Check sheet for the modelled part. Datum: model origin and axes. Units: mm. A direction names the side the tool comes from. Round coordinates to 2 decimals unless told otherwise and drop trailing zeros. Write each loop counter-clockwise with the first axis right and the second up, starting at its lowest first coordinate (ties: lowest second). Pieces come first, ordered by that corner, then holes. Notation, with made-up numbers: (60, 86) - (78, 86) arc R17 ccw to (78, 94) - close; hole circle Ø7 at (30, -13.5). An arc over 180 degrees is marked (long way). Answer as a JSON object with one key per item and string values. Group by question number.
Item 1: Thickness scan on line 1 (Z direction, x = 2.75, y = 73.66) (3 decimals); line 2 (X direction, y = 46, z = -1); line 3 (X direction, y = 39.5, z = 38.5). Record the ranges inside material, lowest first.
Item 2: Gauge pin test, flat ends, axial feed: P1, Ø1.3, axis at x = 1.5, z = -4, coming from the +Y side; P2, Ø5, axis at y = 69.5, z = -1, coming from the +X side; P3, Ø2, axis at x = 1.5, z = 21.5, coming from the +Y side. Record the tip position at first contact, or that the pin passes through.
Item 3: Set-up check for faces 1 (the flat face through (1, 44.45, -28)), 2 (the cylindrical face through (5.633, 81.215, 21.868)): record each of +Z, -Z, +X, -X, +Y, -Y from which the full face is reachable in a straight line by a thin tool's end or side.
Item 4: Sectioned sample at A-A on y = 73.66. Record the boundary of the cut face in (x, z) (3 decimals), plus the area to 3 significant figures.
Item 5: Sectioned sample at B-B on z = 18.5. Record the boundary of the cut face in (x, y).
Item 6: Release check for a two-part mould opening along Z. For faces 3 (the flat face through (5, 63, 50.8)), 4 (the flat face through (6.95, 100.99, 0.71)), 5 (the flat face through (1, 42, 13.511)) record: pulls with the +Z half, pulls with the -Z half, needs draft (parallel to the pull), parting line crosses it, or undercut.
Item 7: Sectioned sample at C-C on x = 6. Record the boundary of the cut face in (y, z) (3 decimals).
Item 8: Sectioned sample at D-D on z = 36. Record the boundary of the cut face in (x, y), plus the area to 3 significant figures.
Autodesk Inventor part; units mm, degrees
ref_plane "YZ Plane" through (0, 0, 0) normal (1, 0, 0) x (0, 1, 0)
ref_plane "XZ Plane" through (0, 0, 0) normal (0, 1, 0) x (-1, 0, 0)
sketch "Sketch1" plane through (0, 0, 0) normal (0, 0, 1) x (1, 0, 0)
  line L0 (0, 0) -> (14.2789, 101.6)
  line L1 (14.2789, 101.6) -> (0, 101.6)
  line L2 (0, 101.6) -> (0, 0)
  dimension "d0" = 101.6
  dimension "d1" = 8
  dimension "d2" = 14.279
extrude "Extrusion1" add sketch "Sketch1" along normal mid plane 101.6
ref_plane "Work Plane2" through (0, 0, 42.3872) normal (-1, 0, 0) x (0, 0, 1)
sketch "Sketch6" plane through (0, 0, 42.3872) normal (-1, 0, 0) x (0, 0, 1)
  line L0 (-84.1061, 73.66) -> (0, 73.66) construction
  line L1 (0, 101.6) -> (0, 0) construction
  line L2 (-84.7743, 101.6) -> (0, 101.6) construction
  circle A0 centre (-65.2472, 73.66) radius 9.525
  circle A1 centre (-19.5272, 73.66) radius 7.62
  line L3 (-42.3872, 121.92) -> (-42.3872, -20.32)
  point P0 (-42.3872, 0)
  dimension "d18" = 27.94
  dimension "d19" = 19.05
  dimension "d20" = 15.24
  dimension "d21" = 22.86
  dimension "d22" = 22.86
  dimension "d23" = 45.72
extrude "Extrusion5" cut sketch "Sketch6" against normal through all
ref_plane "Work Plane3" through (0, 0, 22.86) normal (0, 0, 1) x (1, 0, 0)
ref_plane "Work Plane4" through (0, 0, -22.86) normal (0, 0, 1) x (1, 0, 0)
sketch "Sketch9" plane through (0, 0, -50.8) normal (-1, 0, 0) x (0, 0, 1)
  line L0 (0, 101.6) -> (0, 0) construction
  line L1 (0, 38.1) -> (100.9997, 38.1) construction
  line L2 (0, 0) -> (101.6, 0) construction
  spline S0 degree 2 poles (30.4104, 35.6403) (30.4104, 34.6934) (29.6899, 33.2629) (29.093, 32.7895) knots 0 0 0 1 2 2 2
  spline S1 degree 2 poles (29.093, 32.7895) (28.3726, 32.2234) (26.6642, 31.75) (25.3365, 31.75) knots 0 0 0 1 2 2 2
  line L3 (25.3365, 31.75) -> (20.2627, 31.75)
  line L4 (20.2627, 31.75) -> (20.2627, 44.45)
  line L5 (20.2627, 44.45) -> (24.7396, 44.45)
  spline S2 degree 2 poles (24.7396, 44.45) (26.1393, 44.45) (27.5801, 44.2339) (28.2079, 43.8942) knots 0 0 0 1 2 2 2
  spline S3 degree 2 poles (28.2079, 43.8942) (28.8975, 43.534) (29.5664, 42.299) (29.5664, 41.4963) knots 0 0 0 1 2 2 2
  spline S4 degree 2 poles (29.5664, 41.4963) (29.5664, 40.57) (28.6402, 39.1189) (27.8169, 38.7793) knots 0 0 0 1 2 2 2
  line L6 (27.8169, 38.7793) -> (27.8169, 38.7175)
  spline S5 degree 2 poles (27.8169, 38.7175) (29.0004, 38.4705) (30.4104, 36.937) (30.4104, 35.6403) knots 0 0 0 1 2 2 2
  spline S6 degree 2 poles (27.117, 35.6917) (27.117, 36.2887) (26.6436, 36.9576) (26.1702, 37.1326) knots 0 0 0 1 2 2 2
  spline S7 degree 2 poles (26.1702, 37.1326) (25.882, 37.2458) (24.8631, 37.2664) (24.0192, 37.2664) knots 0 0 0 1 2 2 2
  line L7 (24.0192, 37.2664) -> (23.4326, 37.2664)
  line L8 (23.4326, 37.2664) -> (23.4326, 34.0656)
  line L9 (23.4326, 34.0656) -> (23.6075, 34.0656)
  spline S8 degree 2 poles (23.6075, 34.0656) (24.8425, 34.0656) (25.7894, 34.0965) (26.2834, 34.3126) knots 0 0 0 1 2 2 2
  spline S9 degree 2 poles (26.2834, 34.3126) (26.7156, 34.5082) (27.117, 35.2286) (27.117, 35.6917) knots 0 0 0 1 2 2 2
  spline S10 degree 2 poles (26.3246, 40.8685) (26.3246, 41.1772) (26.0055, 41.8256) (25.6762, 41.9697) knots 0 0 0 1 2 2 2
  spline S11 degree 2 poles (25.6762, 41.9697) (25.3674, 42.1138) (24.5029, 42.1344) (23.6487, 42.1344) knots 0 0 0 1 2 2 2
  line L10 (23.6487, 42.1344) -> (23.4326, 42.1344)
  line L11 (23.4326, 42.1344) -> (23.4326, 39.4379)
  line L12 (23.4326, 39.4379) -> (23.834, 39.4379)
  spline S12 degree 2 poles (23.834, 39.4379) (24.647, 39.4379) (25.3057, 39.4688) (25.6556, 39.6335) knots 0 0 0 1 2 2 2
  spline S13 degree 2 poles (25.6556, 39.6335) (26.0364, 39.8187) (26.3246, 40.4465) (26.3246, 40.8685) knots 0 0 0 1 2 2 2
  line L13 (35.9885, 31.75) -> (40.2801, 44.45)
  line L14 (40.2801, 44.45) -> (43.7587, 44.45)
  line L15 (43.7587, 44.45) -> (48.0504, 31.75)
  line L16 (48.0504, 31.75) -> (44.7673, 31.75)
  line L17 (44.7673, 31.75) -> (43.9749, 34.3435)
  line L18 (43.9749, 34.3435) -> (39.9817, 34.3435)
  line L19 (39.9817, 34.3435) -> (39.1789, 31.75)
  line L20 (39.1789, 31.75) -> (35.9885, 31.75)
  line L21 (43.275, 36.6489) -> (41.9783, 40.8479)
  line L22 (41.9783, 40.8479) -> (40.6712, 36.6489)
  line L23 (40.6712, 36.6489) -> (43.275, 36.6489)
  spline S14 degree 2 poles (60.0094, 31.503) (57.1483, 31.503) (53.7932, 34.961) (53.7932, 38.0897) knots 0 0 0 1 2 2 2
  spline S15 degree 2 poles (53.7932, 38.0897) (53.7932, 41.1052) (57.1586, 44.697) (60.0197, 44.697) knots 0 0 0 1 2 2 2
  spline S16 degree 2 poles (60.0197, 44.697) (60.771, 44.697) (61.9854, 44.522) (62.5412, 44.378) knots 0 0 0 1 2 2 2
  spline S17 degree 2 poles (62.5412, 44.378) (62.9734, 44.2442) (63.9923, 43.8016) (64.3113, 43.637) knots 0 0 0 1 2 2 2
  line L24 (64.3113, 43.637) -> (64.3113, 40.6112)
  line L25 (64.3113, 40.6112) -> (63.9923, 40.6112)
  spline S18 degree 2 poles (63.9923, 40.6112) (63.7556, 40.817) (63.0557, 41.3934) (62.6132, 41.6609) knots 0 0 0 1 2 2 2
  spline S19 degree 2 poles (62.6132, 41.6609) (62.1707, 41.9388) (61.1106, 42.3196) (60.524, 42.3196) knots 0 0 0 1 2 2 2
  spline S20 degree 2 poles (60.524, 42.3196) (59.8344, 42.3196) (58.6921, 41.8874) (58.1672, 41.3419) knots 0 0 0 1 2 2 2
  spline S21 degree 2 poles (58.1672, 41.3419) (57.6938, 40.8582) (57.0865, 39.2012) (57.0865, 38.0794) knots 0 0 0 1 2 2 2
  spline S22 degree 2 poles (57.0865, 38.0794) (57.0865, 36.8959) (57.7143, 35.2801) (58.2289, 34.7861) knots 0 0 0 1 2 2 2
  spline S23 degree 2 poles (58.2289, 34.7861) (58.7229, 34.3024) (59.9374, 33.8804) (60.5446, 33.8804) knots 0 0 0 1 2 2 2
  spline S24 degree 2 poles (60.5446, 33.8804) (61.1724, 33.8804) (62.3147, 34.3024) (62.7058, 34.5596) knots 0 0 0 1 2 2 2
  spline S25 degree 2 poles (62.7058, 34.5596) (63.1381, 34.8169) (63.7865, 35.3624) (64.0232, 35.5785) knots 0 0 0 1 2 2 2
  line L26 (64.0232, 35.5785) -> (64.3113, 35.5785)
  line L27 (64.3113, 35.5785) -> (64.3113, 32.5939)
  spline S26 degree 2 poles (64.3113, 32.5939) (63.9614, 32.4293) (63.0455, 32.0176) (62.5515, 31.8735) knots 0 0 0 1 2 2 2
  spline S27 degree 2 poles (62.5515, 31.8735) (61.9545, 31.6882) (60.9151, 31.503) (60.0094, 31.503) knots 0 0 0 1 2 2 2
  line L28 (82.4351, 31.75) -> (78.5757, 31.75)
  line L29 (78.5757, 31.75) -> (75.128, 36.9062)
  line L30 (75.128, 36.9062) -> (74.5002, 36.0417)
  line L31 (74.5002, 36.0417) -> (74.5002, 31.75)
  line L32 (74.5002, 31.75) -> (71.3097, 31.75)
  line L33 (71.3097, 31.75) -> (71.3097, 44.45)
  line L34 (71.3097, 44.45) -> (74.5002, 44.45)
  line L35 (74.5002, 44.45) -> (74.5002, 38.7793)
  line L36 (74.5002, 38.7793) -> (78.5757, 44.45)
  line L37 (78.5757, 44.45) -> (82.2498, 44.45)
  line L38 (82.2498, 44.45) -> (77.7215, 38.5528)
  line L39 (77.7215, 38.5528) -> (82.4351, 31.75)
  point P0 (50.8, 0)
  dimension "d35" = 38.1
extrude "TextforBack" cut sketch "Sketch9" against normal blind 2.54
sketch "Sketch10" plane through (0, 0, 0) normal (0, 0, 1) x (1, 0, 0)
  line L0 (14.2789, 101.6) -> (0, 0)
  line L1 (0, 101.6) -> (14.2789, 101.6)
  line L2 (0, 0) -> (0, 101.6)
  line L3 (0, 101.6) -> (14.1055, 100.3659)
  line L4 (0, 101.6) -> (14.1594, 101.6) construction
  line L5 (14.1055, 100.3659) -> (14.2789, 101.6)
  line L6 (14.2789, 101.6) -> (0, 101.6)
  dimension "d38" = 5
extrude "Extrusion8" cut sketch "Sketch10" against normal through all both and the other way through all contours L0 L3 L1
properties part number "twoPipeCover"
Completed:
{
 "1": {"line 1": "-50.8 to -32.385, -13.335 to 15.24, 30.48 to 50.8", "line 2": "0 to 6.46", "line 3": "0 to 5.55"},
 "2": {"P1": "y = 101.53", "P2": "x = 10.12", "P3": "y = 101.56"},
 "3": {"face 1": "-X", "face 2": "+X, -X"},
 "4": {"outline": "(0, -50.8) - (10.352, -50.8) - (10.352, -32.385) - (0, -32.385) - close; (0, -13.335) - (10.352, -13.335) - (10.352, 15.24) - (0, 15.24) - close; (0, 30.48) - (10.352, 30.48) - (10.352, 50.8) - (0, 50.8) - close", "area": "697 mm²"},
 "5": {"outline": "(0, 0) - (9.47, 67.41) - (0, 67.41) - close; (0, 79.91) - (11.23, 79.91) - (14.11, 100.37) - (0, 101.6) - close"},
 "6": {"face 3": "pulls with the +Z half", "face 4": "needs draft", "face 5": "undercut"},
 "7": {"outline": "(42.692, -50.8) - (101.075, -50.8) - (101.075, 50.8) - (42.692, 50.8) - close; hole circle Ø19.05 at (73.66, -22.86); hole circle Ø15.24 at (73.66, 22.86)"},
 "8": {"outline": "(0, 0) - (14.11, 100.37) - (0, 101.6) - close", "area": "717 mm²"}
}
